Read the model definition and answer for the solid it produces. Units are mm, in the model's axes. Face numbers are marked on the shaded views. A direction names the side the tool comes from. Give positions to 0.01 mm unless a question says otherwise; leave off trailing zeros. Write each loop counter-clockwise with the first axis right and the second up, starting at its lowest first coordinate (ties: lowest second). Pieces come first, ordered by that corner, then holes. Notation, with made-up numbers: M 26.5,52 L 44.5,52 A8 cw 44.5,61 Z; hole C 63.25,56 d3. An arc over 180 degrees is marked long. Put each result on its own line as item: value.
from build123d import *

# Parameters (mm, degrees)
F0_W      = 55.88
F0_H      = 55.88
F1_DEPTH  = 139.7
F2_R      = 27.93999
F3_W      = 22.4871877581
F3_H      = 35.5748719843
F3_H_2    = 25.40001
F4_DEPTH  = 55.881
F5_R      = 15.24
F6_DEPTH  = 55.881
F7_W      = 84.3253175833
F7_H      = 25.4
F8_DEPTH  = 55.881
F9_R      = 15.2425635054
F10_DEPTH = 55.881


# Not quite as in the source:
# - a fillet or chamfer is up to 0.001 mm smaller than in the source, because OpenCascade refuses the exact size
# - a feature names something its author has since deleted; it is built from what else it names


with BuildPart() as f1:
    # F0 (on Front) → F1 (new body)
    with BuildSketch(Plane.XZ):
        with Locations((27.94, -27.94)):
            Rectangle(F0_W, F0_H)
    extrude(amount=F1_DEPTH)

    # F2 (radius 27.94 in the source; OpenCascade refuses exactly that, so slightly less here)
    f2_edges = [f1.edges().sort_by_distance(p)[0] for p in [
        (0, -139.7, -27.94),
        (27.94, 0, 0),
        (27.94, 0, -55.88),
        (55.88, -139.7, -27.94),
    ]]
    fillet(f2_edges, radius=F2_R)

    # F3 (on face) → F4 (cut, through all)
    with BuildSketch(Plane(origin=(0, 0, -55.88), x_dir=(1, 0, 0), z_dir=(0, 0, -1))):
        with Locations((29.396406121, 10.1525540079)):
            Rectangle(F3_W, F3_H)
        with Locations((29.396406121, 40.639995)):
            Rectangle(F3_W, F3_H_2)
    extrude(amount=-F4_DEPTH, mode=Mode.SUBTRACT)

    # F5 (on face) → F6 (cut, through all)
    with BuildSketch(Plane(origin=(0, 0, 0), x_dir=(0, -1, 0), z_dir=(-1, 0, 0))):
        with Locations((27.94, -27.94)):
            Circle(F5_R)
    extrude(amount=-F6_DEPTH, mode=Mode.SUBTRACT)

    # F7 (on face) → F8 (cut, through all)
    with BuildSketch(Plane(origin=(0, 0, 0), x_dir=(0, -1, 0), z_dir=(-1, 0, 0))):
        with Locations((128.5226587916, -27.94)):
            Rectangle(F7_W, F7_H)
    extrude(amount=-F8_DEPTH, mode=Mode.SUBTRACT)

    # F9 (on face) → F10 (cut, through all)
    with BuildSketch(Plane(origin=(0, 0, -55.88), x_dir=(1, 0, 0), z_dir=(0, 0, -1))):
        with Locations((27.94, 111.76)):
            Circle(F9_R)
    extrude(amount=-F10_DEPTH, mode=Mode.SUBTRACT)


solid = f1.part
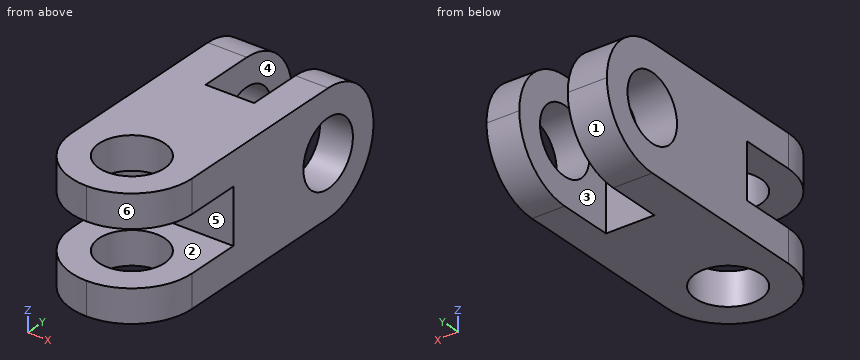
(1) Given pin 1 Ø1.5 at (x, z) = (29, -50) entering from +Y; pin 2 Ø1.5 at (y, z) = (-115, -48.5) entering from +X; pin 3 Ø3 at (x, z) = (10.5, -10.5) entering from +Y; pin 4 Ø24.5 at (x, y) = (27.94, -111.76) entering from -Z, each flat-ended and moving along its own axis, determine where each tip first touches the part or whether it passes through.
Result:
pin 1: stops at y = -53.34
pin 2: stops at x = 55.77
pin 3: stops at y = -4.99
pin 4: passes through
(2) Section A-A on y = -44.5 is taken. Determine the outline of the cut face in (x, z), and give its area (3 significant figures).
Result:
outline: M 0,-55.88 L 18.15,-55.88 L 18.15,0 L 0,0 Z; M 40.64,-55.88 L 55.88,-55.88 L 55.88,0 L 40.64,0 Z
area: 1,870 mm²
(3) Section B-B on z = -35.5 is taken. Determine the outline of the cut face in (x, y).
Result:
outline: M 0,-86.36 L 55.88,-86.36 L 55.88,-41.17 L 40.64,-41.17 L 40.64,-53.34 L 18.15,-53.34 L 18.15,-41.17 L 0,-41.17 Z; M 0,-14.71 L 18.15,-14.71 L 18.15,-1.04 L 0,-1.04 Z; M 40.64,-14.71 L 55.88,-14.71 L 55.88,-1.04 L 40.64,-1.04 Z
(4) For a pull along X with two mould halves and no side action, classify the marked faces 4, 5 and 6 as +X half, -X half, draft (parallel to the pull), parting line (faces both ways), or undercut.
Result:
face 4: undercut
face 5: draft
face 6: +X half
(5) Which of the six approach directions +Z, -Z, +X, -X, +Y, -Y give full straight-line access (tool end or side, diameter ignored) to the marked faces 1, 2 and 3?
Result:
face 1: -Z, +X, -X, +Y
face 2: +X, -X, -Y
face 3: +Z, -Z, +Y
(6) Straight lines are drawn through the part: line 1 along Z through (x, y) = (50, -103); line 2 along X through (y, z) = (-18, -43); line 3 along Z through (x, y) = (49, -27). For each, find the intervals that lie inside material, in ascending order. Write a range as from..to.
Result:
line 1: z = -55.88..-40.64, -15.24..0
line 2: x = 0..18.15, 40.64..55.88
line 3: z = -55.86..-43.15, -12.73..-0.02
(7) Section D-D on y = -21 is taken. Determine the outline of the cut face in (x, z), and give its area (3 significant figures).
Result:
outline: M 0,-55 L 18.15,-55 L 18.15,-41.51 L 0,-41.51 Z; M 0,-14.37 L 18.15,-14.37 L 18.15,-0.88 L 0,-0.88 Z; M 40.64,-55 L 55.88,-55 L 55.88,-41.51 L 40.64,-41.51 Z; M 40.64,-14.37 L 55.88,-14.37 L 55.88,-0.88 L 40.64,-0.88 Z
area: 901 mm²
